Check sheet for the modelled part. Datum: model origin and axes. Units: mm. Face numbers are marked on the shaded views. A direction names the side the tool comes from. Round coordinates to 2 decimals unless told otherwise and drop trailing zeros. Order: outer loops, then holes, each group sorted by start corner. A loop starts at its lowest first (then second) coordinate and runs counter-clockwise, first axis right, second up.
(1) Sectioned sample at C-C, the plane x = 0. Enter the section's corners in (y, z), and give its area (3 significant figures).
(2) Mould release check, pull along X, two halves, no side actions. Record for the marked faces 1, 2 and 3: released by +X, released by -X, zero draft, split by the parting line, or undercut.
(3) Depth check by flat-ended pin: pin 1 (1.8 mm diameter, centred on x = -2, y = 16, fed in from +Z); pin 2 (2 mm diameter, centred on x = 2.5, y = -11.5, fed in from +Z); pin 3 (1.5 mm diameter, centred on x = -5.5, z = 0, fed in from -Y). Enter the tip coordinate at first touch or a pass-through.
(4) Thickness scan on probe 1 along Y at (x, z) = (0, 4); probe 2 along Z at (x, y) = (2, 13); probe 3 along X at (y, z) = (0, 2.5). Record the ranges inside material, lowest first.
(5) Sectioned sample at B-B, the plane y = 0. Enter the section's corners in (x, z), and give its area (3 significant figures).
(6) Sectioned sample at A-A, the plane z = -1. Enter the section's corners in (x, y), and give its area (3 significant figures).
(7) Sectioned sample at D-D, the plane z = 5.5. Enter the section's corners in (x, y).
(8) Tool access check on the marked faces 4, 5, 6, 7 and 8. Record the directions out of +Z, -Z, +X, -X, +Y, -Y that give a thin tool (end or side, any length) a straight path to the whole face; none if there is none.
```python
from build123d import *

# Parameters (mm, degrees)
BOSS_EXTRUDE1_DEPTH     = 8
CUT_EXTRUDE1_DEPTH      = 26.124689053
CUT_EXTRUDE1_DEPTH_BACK = 26.124689053
SKETCH2_R               = 4


with BuildPart() as part:
    # Sketch1 → Boss-Extrude1 (new, symmetric)
    with BuildSketch(Plane.YZ):
        with BuildLine():
            Line((8, 9), (-8, 9))
            ThreePointArc((-8, 9), (-9.843962907, 6.816699867), (-12.582575695, 6))
            Line((-12.582575695, 6), (-18.5, 6))
            Line((-18.5, 6), (-18.5, 2))
            Line((-18.5, 2), (-12.5, 2))
            Line((-12.5, 2), (-12.5, -2))
            Line((-12.5, -2), (-18.5, -2))
            Line((-18.5, -2), (-18.5, -6))
            Line((-18.5, -6), (-8.5, -6))
            Line((-8.5, -6), (-8.5, 0))
            Line((-8.5, 0), (8.5, 0))
            Line((8.5, 0), (8.5, -6))
            Line((8.5, -6), (18.5, -6))
            Line((18.5, -6), (18.5, -2))
            Line((18.5, -2), (12.5, -2))
            Line((12.5, -2), (12.5, 2))
            Line((12.5, 2), (18.5, 2))
            Line((18.5, 2), (18.5, 6))
            Line((18.5, 6), (12.582575695, 6))
            ThreePointArc((12.582575695, 6), (9.843962907, 6.816699867), (8, 9))
        make_face()
    extrude(amount=BOSS_EXTRUDE1_DEPTH, both=True)

    # Sketch2 → Cut-Extrude1 (cut, two sides: drawn at the far end of the back side and taken through both)
    with BuildSketch(Plane.XY.offset(9).offset(-CUT_EXTRUDE1_DEPTH_BACK)):
        Circle(SKETCH2_R)
    extrude(amount=CUT_EXTRUDE1_DEPTH + CUT_EXTRUDE1_DEPTH_BACK, mode=Mode.SUBTRACT)


solid = part.part
```
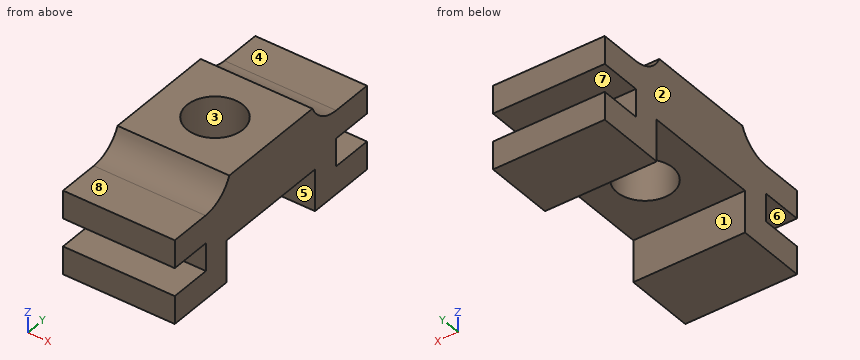
Derived:
1. outline: (-18.5, -6) - (-8.5, -6) - (-8.5, 0) - (-4, 0) - (-4, 9) - (-8, 9) arc R5 cw to (-12.58, 6) - (-18.5, 6) - (-18.5, 2) - (-12.5, 2) - (-12.5, -2) - (-18.5, -2) - close; (4, 0) - (8.5, 0) - (8.5, -6) - (18.5, -6) - (18.5, -2) - (12.5, -2) - (12.5, 2) - (18.5, 2) - (18.5, 6) - (12.58, 6) arc R5 cw to (8, 9) - (4, 9) - close
1. area: 278 mm2
2. face 1: zero draft
2. face 2: released by -X
2. face 3: undercut
3. pin 1: stops at z = 6
3. pin 2: stops at z = 6.45
3. pin 3: stops at y = -12.5
4. probe 1: y = -18.5 to -4, 4 to 18.5
4. probe 2: z = -6 to -2, 2 to 6
4. probe 3: x = -8 to -4, 4 to 8
5. outline: (-8, 0) - (-4, 0) - (-4, 9) - (-8, 9) - close; (4, 0) - (8, 0) - (8, 9) - (4, 9) - close
5. area: 72.0 mm2
6. outline: (-8, -12.5) - (8, -12.5) - (8, -8.5) - (-8, -8.5) - close; (-8, 8.5) - (8, 8.5) - (8, 12.5) - (-8, 12.5) - close
6. area: 128 mm2
7. outline: (-8, -18.5) - (8, -18.5) - (8, 18.5) - (-8, 18.5) - close; hole circle Ø8 at (0, 0)
8. face 4: +Z, +X, -X, +Y
8. face 5: -Z, +X, -X
8. face 6: +X, -X, -Y
8. face 7: +X, -X, +Y
8. face 8: +Z, +X, -X, -Y
